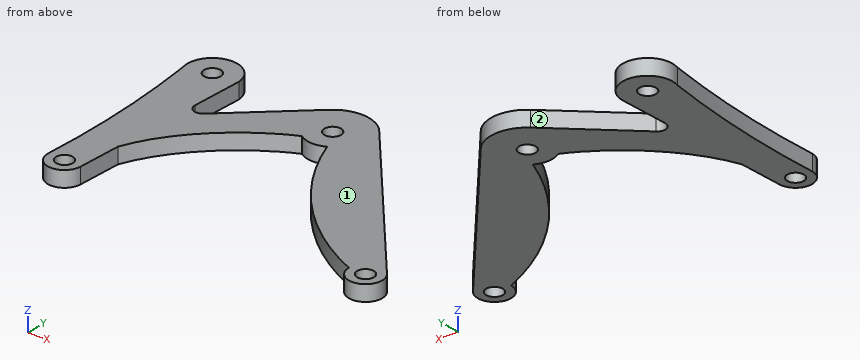
Autodesk Inventor part; units mm, degrees
ref_plane "YZ Plane" through (0, 0, 0) normal (1, 0, 0) x (0, 1, 0)
ref_plane "XZ Plane" through (0, 0, 0) normal (0, 1, 0) x (-1, 0, 0)
ref_plane "XY Plane" through (0, 0, 0) normal (0, 0, 1) x (1, 0, 0)
sketch "Sketch1" plane through (0, 0, 0) normal (0, 0, 1) x (1, 0, 0)
  line L0 (-110, 70) -> (110, 70) construction
  line L1 (110, 70) -> (110, -70) construction
  line L2 (110, -70) -> (-110, -70) construction
  line L3 (-110, -70) -> (-110, 70) construction
  circle A0 centre (-90, 55) radius 5
  circle A1 centre (-90, -55) radius 5
  circle A2 centre (90, -55) radius 5
  circle A3 centre (-10, 45) radius 5
  line L4 (-67, 0) -> (-42, 0) construction
  line L5 (-42, 0) -> (-42, -30) construction
  line L6 (-42, -30) -> (-67, -30) construction
  line L7 (-67, -30) -> (-67, 0) construction
  circle A4 centre (-54.5, -19) radius 10 construction
  arc A5 (-75.0363, 56.0433) -> (-104.3936, 50.7781) centre (-90, 55) ccw
  arc A6 (-99.9402, -53.9078) -> (-80.0103, -55.4531) centre (-90, -55) ccw
  arc A7 (-100, -55) -> (-105, 55) centre (-644.4063, -24.6321) ccw
  line L8 (-78.8103, -29) -> (-67, 2.1947) construction
  line L9 (-67, 2.1947) -> (-37.7539, 24.0313) construction
  line L10 (-37.7539, 24.0313) -> (-18.5252, 32.6582) construction
  spline S0 degree 3 poles (-78.8103, -29) (-67, 2.1947) (-37.7539, 24.0313) (-18.5252, 32.6582) knots 1 1 1 1 2 2 2 2
  line L11 (-24.7333, 61.0503) -> (-68.0357, 21.3009)
  line L12 (-75.0363, 56.0433) -> (-76.412, 25.2072)
  line L13 (-78.8103, -29) -> (-80.0103, -55.4531)
  arc A8 (80, -55) -> (97.6312, -48.5374) centre (90, -55) ccw
  line L14 (5.1977, 60.6112) -> (97.6312, -48.5374)
  arc A9 (-2.7947, 31.8439) -> (80, -55) centre (141.6446, 86.6595) ccw
  arc A10 (-18.5252, 32.6582) -> (-2.7947, 31.8439) centre (-10, 45) ccw
  arc A11 (5.1977, 60.6112) -> (-24.7333, 61.0503) centre (-10, 45) ccw
  arc A12 (-76.412, 25.2072) -> (-68.0357, 21.3009) centre (-71.4169, 24.9844) ccw
  point P0 (0, 0)
  dimension "d1" = 70
  dimension "d2" = 70
  dimension "d3" = 110
  dimension "d4" = 110
  dimension "d5" = 10
  dimension "d6" = 10
  dimension "d7" = 10
  dimension "d8" = 10
  dimension "d9" = 55
  dimension "d10" = 55
  dimension "d11" = 55
  dimension "d12" = 180
  dimension "d13" = 90
  dimension "d15" = 10
  dimension "d16" = 45
  dimension "d17" = 42
  dimension "d18" = 30
  dimension "d19" = 0
  dimension "d20" = 25
  dimension "d21" = 20
  dimension "d25" = 19
  dimension "d26" = 12.5
  dimension "d67" = 90
  dimension "d68" = 30
  dimension "d70" = 20
  dimension "d71" = 20
  dimension "d74" = 10
extrude "Extrusion6" add sketch "Sketch1" along normal blind 9.4 contours L12 A12 L11 A11 L14 A8 A9 A10 S0 L13 A6 A7 A5 | A7 A5
equation "\"d26\" = 0.5 * d20"
properties part number "Bracket Concept MK8"
Verification items for the finished model (mm, model axes). Face numbers are marked on the shaded views. Coordinates: 2 decimals unless noted, no trailing zeros. Write each loop counter-clockwise with the first axis right and the second up, starting at its lowest first coordinate (ties: lowest second). Pieces come first, ordered by that corner, then holes. Notation, with made-up numbers: M 44.25,52.5 L 50.25,52.5 A19 cw 50.25,78.5 Z; hole C 72,-4.75 d9. An arc over 180 degrees is marked long. Answer as a JSON object with one key per item and string values. Group by question number.
(1) Cross-section at C-C, the plane x = -90. Record the cut outline in (y, z).
(2) Cross-section at A-A, the plane x = -10. Record the cut outline in (y, z).
(3) Gauge pin test, flat ends, axial feed: pin 1 (5 mm diameter, centred on x = -1.5, z = 2, fed in from +Y); pin 2 (6 mm diameter, centred on x = -90, y = -55, fed in from +Z); pin 3 (5 mm diameter, centred on y = 1, z = 7, fed in from +X); pin 4 (1 mm diameter, centred on x = 59, z = 8, fed in from -Y). Record the tip position at first contact, or that the pin passes through.
(4) Material ranges on line 1 (Y direction, x = -90, z = 2.5); line 2 (X direction, y = 27, z = 1); line 3 (X direction, y = 11, z = 4.25), recorded low to high.
(5) Cross-section at D-D, the plane y = 45. Record the cut outline in (x, z), and give its area (3 significant figures).
(6) Release check for a two-part mould opening along X. For the marked faces 1 and 2 record: +X half, -X half, draft (parallel to the pull), parting line (faces both ways), or undercut.
(7) Cross-section at B-B, the plane y = -46. Record the cut outline in (x, z), and give its area (3 significant figures).
Reply:
{
 "1": {"outline": "M -65,0 L -60,0 L -60,9.4 L -65,9.4 Z; M -50,0 L 50,0 L 50,9.4 L -50,9.4 Z; M 60,0 L 70,0 L 70,9.4 L 60,9.4 Z"},
 "2": {"outline": "M 30,0 L 40,0 L 40,9.4 L 30,9.4 Z; M 50,0 L 66.79,0 L 66.79,9.4 L 50,9.4 Z"},
 "3": {"pin 1": "y = 65.94", "pin 2": "through", "pin 3": "x = 57.8", "pin 4": "y = -44.18"},
 "4": {"line 1": "-65 to -60, -50 to 50, 60 to 70", "line 2": "-101.6 to -76.33, -61.83 to -29.29, -0.86 to 33.66", "line 3": "-100.32 to -50.68, 6.95 to 47.21"},
 "5": {"outline": "M -103.62,0 L -75.53,0 L -75.53,9.4 L -103.62,9.4 Z; M -42.22,0 L -15,0 L -15,9.4 L -42.22,9.4 Z; M -5,0 L 18.42,0 L 18.42,9.4 L -5,9.4 Z", "area": "740 mm²"},
 "6": {"face 1": "draft", "face 2": "undercut"},
 "7": {"outline": "M -99.57,0 L -79.58,0 L -79.58,9.4 L -99.57,9.4 Z; M 62.47,0 L 95.48,0 L 95.48,9.4 L 62.47,9.4 Z", "area": "498 mm²"}
}
